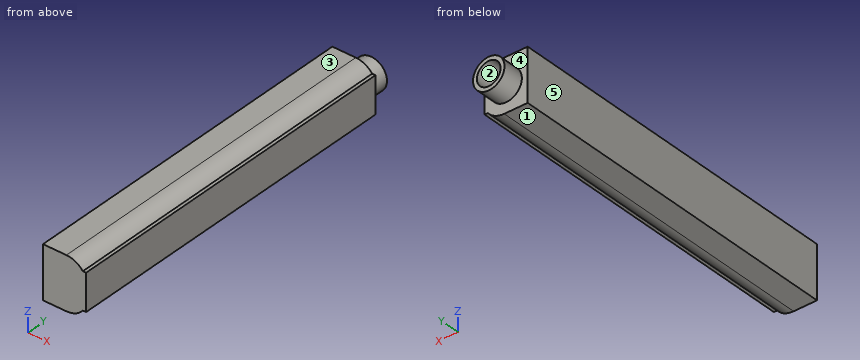
from build123d import *

# Parameters (mm, degrees)
BOSS_EXTRUDE1_DEPTH = 1.5
BOSS_EXTRUDE2_START = 131.6
BOSS_EXTRUDE2_DEPTH = 131.6
BOSS_EXTRUDE3_DEPTH = 1.5
SKETCH4_R           = 6
SKETCH4_R_2         = 4.5
BOSS_EXTRUDE4_DEPTH = 8
CUT_EXTRUDE2_START  = -8
SKETCH6_R           = 4.5
CUT_EXTRUDE2_DEPTH  = 8


with BuildPart() as part:
    # Sketch1 → Boss-Extrude1 (new body)
    with BuildSketch(Plane(origin=(0, 0, 0), x_dir=(1, 0, 0), z_dir=(0, 1, 0))):
        with BuildLine():
            Line((-16.414997998, 3), (-16.414997998, -17))
            Line((-16.414997998, -17), (-7.484997998, -17))
            ThreePointArc((-7.484997998, -17), (-4.020896383, -16.211102551), (-1.24, -14))
            Line((-1.24, -14), (0, -14))
            Line((0, -14), (0, 0))
            Line((0, 0), (-1.24, 0))
            ThreePointArc((-1.24, 0), (-4.020896383, 2.211102551), (-7.484997998, 3))
            Line((-7.484997998, 3), (-16.414997998, 3))
        make_face()
    extrude(amount=-BOSS_EXTRUDE1_DEPTH)

    # Sketch2 → Boss-Extrude2 (add)
    with BuildSketch(Plane(origin=(0, 0, 0), x_dir=(1, 0, 0), z_dir=(0, 1, 0)).offset(BOSS_EXTRUDE2_START)):
        with BuildLine():
            Line((-16.414997998, 3), (-16.414997998, -17))
            Line((-16.414997998, -17), (-7.484997998, -17))
            ThreePointArc((-7.484997998, -17), (-4.020896383, -16.211102551), (-1.24, -14))
            Line((-1.24, -14), (0, -14))
            Line((0, -14), (0, 0))
            Line((0, 0), (-1.24, 0))
            ThreePointArc((-1.24, 0), (-4.020896383, 2.211102551), (-7.484997998, 3))
            Line((-7.484997998, 3), (-16.414997998, 3))
        make_face()
        with BuildLine():
            Line((-7.484997998, 1.5), (-14.914997998, 1.5))
            Line((-14.914997998, 1.5), (-14.914997998, -15.5))
            Line((-14.914997998, -15.5), (-7.484997998, -15.5))
            ThreePointArc((-7.484997998, -15.5), (-4.362498999, -14.700877125), (-2.007772423, -12.5))
            Line((-2.007772423, -12.5), (-1.5, -12.5))
            Line((-1.5, -12.5), (-1.5, -1.5))
            Line((-1.5, -1.5), (-2.007772423, -1.5))
            ThreePointArc((-2.007772423, -1.5), (-4.362498999, 0.700877125), (-7.484997998, 1.5))
        make_face(mode=Mode.SUBTRACT)
    extrude(amount=-BOSS_EXTRUDE2_DEPTH)

    # Sketch3 → Boss-Extrude3 (add)
    with BuildSketch(Plane(origin=(0, 131.6, 0), x_dir=(1, 0, 0), z_dir=(0, 1, 0))):
        with BuildLine():
            Line((-7.484997998, 3), (-16.414997998, 3))
            Line((-16.414997998, 3), (-16.414997998, -17))
            Line((-16.414997998, -17), (-7.484997998, -17))
            ThreePointArc((-7.484997998, -17), (-4.020896383, -16.211102551), (-1.24, -14))
            Line((-1.24, -14), (0, -14))
            Line((0, -14), (0, 0))
            Line((0, 0), (-1.24, 0))
            ThreePointArc((-1.24, 0), (-4.020896383, 2.211102551), (-7.484997998, 3))
        make_face()
    extrude(amount=-BOSS_EXTRUDE3_DEPTH)

    # Sketch4 → Boss-Extrude4 (add)
    with BuildSketch(Plane(origin=(0, 131.6, 0), x_dir=(1, 0, 0), z_dir=(0, 1, 0))):
        with Locations(Location((-8.207498999, -6.780386744, 0), (0, 0, 270))):
            Circle(SKETCH4_R)
        with Locations(Location((-8.207498999, -6.780386744, 0), (0, 0, 270))):
            Circle(SKETCH4_R_2, mode=Mode.SUBTRACT)
    extrude(amount=BOSS_EXTRUDE4_DEPTH)

    # Sketch6 → Cut-Extrude2 (cut)
    with BuildSketch(Plane(origin=(0, 131.6, 0), x_dir=(1, 0, 0), z_dir=(0, 1, 0)).offset(CUT_EXTRUDE2_START)):
        with Locations(Location((-8.207498999, -6.780386744, 0), (0, 0, 270))):
            Circle(SKETCH6_R)
    extrude(amount=CUT_EXTRUDE2_DEPTH, mode=Mode.SUBTRACT)


solid = part.part
Read the model definition and answer for the solid it produces. Units are mm, in the model's axes. Face numbers are marked on the shaded views. A direction names the side the tool comes from. Coordinates: 2 decimals unless noted, no trailing zeros. Loops run counter-clockwise (first coordinate to the right, second up) from the corner with the lowest first, then second, coordinate; pieces in that order, holes last.
Q1. The part is cut by section C-C on z = 5.25. Write down the section's boundary in (x, y) (3 decimals).
Q2. The part is cut by section B-B on x = -11.5. Write down the section's boundary in (y, z).
Q3. The mould has two halves that part along Z. Classify the marked faces 1, 2 and 3: +Z half, -Z half, draft (parallel to the pull), parting line (faces both ways), or undercut.
Q4. This flat-tipped pin is pushed along its axis until it touches: pin 1 Ø8 at (x, z) = (-4, 7) entering from +Y. Where does it stop, or does it pass through?
Q5. The part is cut by section A-A on y = 84.5. Write down the section's boundary in (x, z) (3 decimals), and give its area (3 significant figures).
Q6. Consider probe 1 along Y at (x, z) = (-3.25, 7.5); probe 2 along Z at (x, y) = (-10, 42); probe 3 along X at (y, z) = (54, 9.25) (3 decimals). Determine where each line is inside the solid, lowest interval first.
Q7. Which of the six approach directions +Z, -Z, +X, -X, +Y, -Y give full straight-line access (tool end or side, diameter ignored) to the marked faces 4 and 5?
Results below:
1. outline: (-16.415, -1.5) - (0, -1.5) - (0, 131.6) - (-2.406, 131.6) - (-2.406, 139.6) - (-3.976, 139.6) - (-3.976, 130.1) - (-1.5, 130.1) - (-1.5, 0) - (-14.915, 0) - (-14.915, 130.1) - (-12.439, 130.1) - (-12.439, 139.6) - (-14.009, 139.6) - (-14.009, 131.6) - (-16.415, 131.6) - close
2. outline: (-1.5, -3) - (131.6, -3) - (131.6, 1.76) - (139.6, 1.76) - (139.6, 3.71) - (130.1, 3.71) - (130.1, -1.5) - (0, -1.5) - (0, 15.5) - (130.1, 15.5) - (130.1, 9.85) - (139.6, 9.85) - (139.6, 11.8) - (131.6, 11.8) - (131.6, 17) - (-1.5, 17) - close
3. face 1: -Z half
3. face 2: undercut
3. face 3: +Z half
4. pin 1: stops at y = 139.6
5. outline: (-16.415, -3) - (-7.485, -3) arc R8 ccw to (-1.24, 0) - (0, 0) - (0, 14) - (-1.24, 14) arc R8 ccw to (-7.485, 17) - (-16.415, 17) - close; hole (-14.915, -1.5) - (-7.485, -1.5) arc R6.5 ccw to (-2.008, 1.5) - (-1.5, 1.5) - (-1.5, 12.5) - (-2.008, 12.5) arc R6.5 ccw to (-7.485, 15.5) - (-14.915, 15.5) - close
5. area: 94.2 mm2
6. probe 1: y = -1.5 to 0, 130.1 to 139.6
6. probe 2: z = -3 to -1.5, 15.5 to 17
6. probe 3: x = -16.415 to -14.915, -1.5 to 0
7. face 4: +Y
7. face 5: +Z, -Z, -X, +Y, -Y
